Design review of the part shown in the three views and the two pictorial views. Dimensions are in mm from the part's minimum x, y and z. Give positions to 0.01 mm unless a question says otherwise; leave off trailing zeros. Loops run counter-clockwise (first coordinate to the right, second up) from the corner with the lowest first, then second, coordinate; pieces in that order, holes last. Notation, with made-up numbers: (26, 33) -> (51, 33) arc R23 ccw to (51, 71) -> close; hole circle Ø8 at (42.25, -2). An arc over 180 degrees is marked (long way). One line per question, with ' | ' between items. Start each with the question number.
(1) Insertion check: P1, Ø1.5, axis at x = 28, y = 13.5, coming from the +Z side; P2, Ø4, axis at x = 31, y = 5, coming from the -Z side; P3, Ø1, axis at y = 4, z = 0.5, coming from the -X side (1 decimal); P4, Ø1, axis at y = 22.5, z = 1.5, coming from the +X side. Each pin has a flat end and moves straight along its axis. Give the tip position at first contact, or say it passes through.
(2) Consider section A-A (z = 2.1). Give the number of separate pieces and of enclosed holes in the cut face, and give its area (3 significant figures).
(3) Consider section D-D (x = 17.5). Write out the cut boundary in (y, z).
(4) Wall thickness on probe 1 along Y at (x, z) = (6.5, 2.2) (1 decimal); probe 2 along X at (y, z) = (23, 2.35) (1 decimal); probe 3 along Z at (x, y) = (7, 20.5): over which ranges is each line inside the solid? List them lowest first.
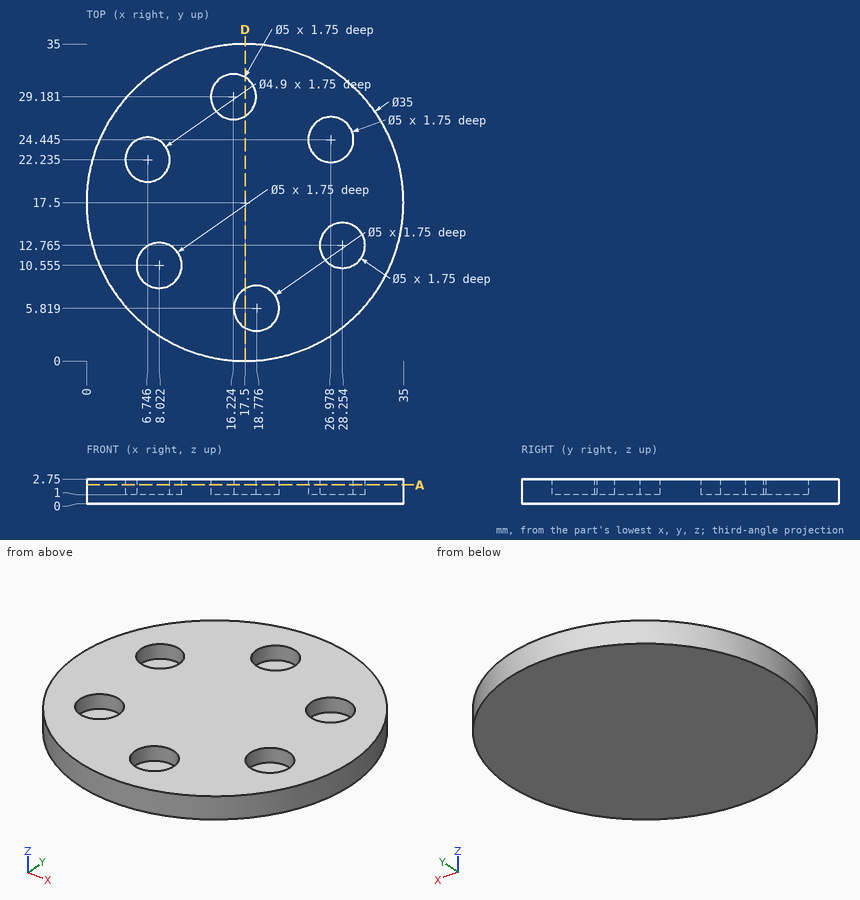
A:
1) P1: stops at z = 1 | P2: stops at z = 0 | P3: stops at x = 5.8 | P4: stops at x = 34.41
2) separate pieces: 1 | enclosed holes: 6 | area: 845 mm^2
3) outline: (0, 0) -> (35, 0) -> (35, 2.75) -> (31.33, 2.75) -> (31.33, 1) -> (27.03, 1) -> (27.03, 2.75) -> (7.97, 2.75) -> (7.97, 1) -> (3.67, 1) -> (3.67, 2.75) -> (0, 2.75) -> close
4) probe 1: y = 3.9 to 8.6, 12.5 to 19.8, 24.7 to 31.1 | probe 2: x = 0.9 to 4.4, 9.1 to 24.9, 29 to 34.1 | probe 3: z = 0 to 1
